Design review of the part built by this model. Coordinates are the model's own, in mm. A direction names the side the tool comes from. Coordinates: 2 decimals unless noted, no trailing zeros. Order: outer loops, then holes, each group sorted by start corner. A loop starts at its lowest first (then second) coordinate and runs counter-clockwise, first axis right, second up. Notation, with made-up numbers: (-23, 87) - (-1, 87) arc R38 ccw to (-1, 125) - close; hole circle Ø2 at (13.5, -12). An arc over 180 degrees is marked (long way). Write item = value, one per line. Start each with the question number.
Solid Edge part; units mm, degrees
sketch "Sketch1" plane through (0, 0, 0) normal (0, 0, 1) x (1, 0, 0)
  circle A0 centre (0, 0) radius 101.5
extrude "Protrusion1" add sketch "Sketch1" along normal blind 19
sketch "Sketch2" plane through (0, 0, 19) normal (0, 0, 1) x (1, 0, 0)
  circle A0 centre (0.4019, -85.9991) radius 8
extrude "ExtrudedCutout_1" cut sketch "Sketch2" along normal mid plane 72.3819
pattern_circular "Pattern1" count 6 over 360 about axis through (0, 0, 19) along (0, 0, -1) of "ExtrudedCutout_1"
sketch "Sketch3" plane through (0, 0, 19) normal (0, 0, 1) x (1, 0, 0)
  circle A0 centre (0, 0) radius 32
extrude "ExtrudedProtrusion_3" add sketch "Sketch3" along normal blind 51
sketch "Sketch4" plane through (0, 0, 70) normal (0, 0, 1) x (0, 1, 0)
  circle A0 centre (0, 0) radius 16
extrude "ExtrudedCutout_3" cut sketch "Sketch4" along normal mid plane 382.6362
sketch "Sketch5" plane through (0, 0, 0) normal (0, -1, 0) x (1, 0, 0)
  line L0 (32, 70) -> (123.9402, 36.8752)
  line L1 (101.5, 0) -> (117.5, 0)
  line L2 (0, 0) -> (101.5, 0)
  line L3 (0, 70) -> (0, 0)
  line L4 (32, 70) -> (0, 70)
  arc A0 (123.9402, 36.8752) -> (117.5, 0) centre (117.5, 19) cw
  circle A1 centre (117.5, 19) radius 6.5
extrude "ExtrudedProtrusion_6" add sketch "Sketch5" along normal mid plane 16
pattern_circular "Pattern3" count 3 over 360 about axis through (0, 0, 19) along (0, 0, -1) of "ExtrudedProtrusion_6"
sketch "Sketch6" plane through (0, 0, 70) normal (0, 0, 1) x (0, 1, 0)
  circle A0 centre (0, 0) radius 16
extrude "ExtrudedCutout_4" cut sketch "Sketch6" along normal mid plane 1270.4141
Item 1: Add section A-A on y = 0. Give the boundary of the cut face in (x, z), plus the area to 3 significant figures.
Item 2: Add section B-B on x = 0. Give the boundary of the cut face in (y, z).
Item 3: Add section C-C on z = 61.5. Give the boundary of the cut face in (x, y), plus the area to 3 significant figures.
Item 4: For faces 1 (the flat face through (84, -8, 35)), 2 (the cylindrical face through (-32, 0, 44)), 3 (the flat face through (84, 8, 35)), 4 (the flat face through (-18, 1, 0)), 5 (the cylindrical face through (-66.284, -43.699, 9.633)), list the 3-axis set-ups (+Z, -Z, +X, -X, +Y, -Y) from which the entire face can be reached by the end or side of a thin tool; tool diameter is ignored.
Item 5: Add section D-D on y = 39. Give the boundary of the cut face in (x, z).
Item 6: Mouldability with a two-part tool opening along Z and no side actions: class faces 6 (the cylindrical face through (14.195, 7.383, 35.49)), 7 (the flat face through (-38.57, -67.02, 53.67)), 8 (the cylindrical face through (-55.41, -96.19, 18.71)) as +Z half, -Z half, draft (parallel to the pull), parting line (faces both ways), or undercut.
Item 7: For line 1 (Y direction, x = 71.5, z = 26); line 2 (Z direction, x = -56.5, y = -2.5); line 3 (X direction, y = 0, z = 30), list the stretches that pass through material, from the lowest coordinate up.
Item 8: For P1, Ø21, axis at x = -0.4, y = 86, coming from the +Z side; P2, Ø4, axis at y = 52, z = 30.5, coming from the -X side; P3, Ø1, axis at y = 74, z = 44.5, coming from the +X side; P4, Ø21, axis at x = -74.68, y = 42.65, coming from the -Z side, all flat-tipped, find the tip position at first contact; note any pin that passes through.
Worked out:
q1.outline = (-101.5, 0) - (-16, 0) - (-16, 70) - (-32, 70) - (-32, 19) - (-101.5, 19) - close; (16, 0) - (117.5, 0) arc R19 ccw to (123.94, 36.88) - (32, 70) - (16, 70) - close; hole circle Ø13 at (117.5, 19)
q1.area = 8,670 mm2
q2.outline = (-101.5, 0) - (-93.99, 0) - (-93.99, 19) - (-101.5, 19) - close; (-78.01, 0) - (-16, 0) - (-16, 70) - (-32, 70) - (-32, 19) - (-78.01, 19) - close; (16, 0) - (78.01, 0) - (78.01, 19) - (32, 19) - (32, 70) - (16, 70) - close; (93.99, 0) - (101.5, 0) - (101.5, 19) - (93.99, 19) - close
q3.outline = (-34.72, -44.14) - (-20.87, -52.14) - (-8.56, -30.83) arc R32 ccw to (30.98, -8) - (55.59, -8) - (55.59, 8) - (30.98, 8) arc R32 ccw to (-8.56, 30.83) - (-20.87, 52.14) - (-34.72, 44.14) - (-22.42, 22.83) arc R32 ccw to (-22.42, -22.83) - close; hole circle Ø32 at (0, 0)
q3.area = 3,560 mm2
q4.face_1 = +Z, +X, -Y
q4.face_2 = +Z, -X
q4.face_3 = +Z, +X, +Y
q4.face_4 = -Z, +X, -X, +Y, -Y
q4.face_5 = +Z, -Z
q5.outline = (-93.71, 0) - (-81.8, 0) - (-81.8, 19) - (-93.71, 19) - close; (-67.56, 0) - (67.56, 0) - (67.56, 19) - (-13.28, 19) - (-13.28, 66.97) - (-31.75, 63.64) - (-31.75, 19) - (-67.56, 19) - close; (80.99, 0) - (93.71, 0) - (93.71, 19) - (80.99, 19) - close
q6.face_6 = draft
q6.face_7 = +Z half
q6.face_8 = undercut
q7.line_1 = -8 to 8
q7.line_2 = 0 to 19
q7.line_3 = -32 to -16, 16 to 132.99
q8.P1 = 19
q8.P2 = -40.41
q8.P3 = -33.2
q8.P4 = 0
